```python
from build123d import *

# Parameters (mm, degrees)
SKETCH1_W           = 50
SKETCH1_H           = 170
BOSS_EXTRUDE1_DEPTH = 55
SKETCH2_W           = 34
SKETCH2_H           = 27
CUT_EXTRUDE1_DEPTH  = 181.416185527
SKETCH3_W           = 10
SKETCH3_H           = 24
SKETCH3_R           = 4.25
SKETCH3_R_2         = 1
CUT_EXTRUDE2_DEPTH  = 186.539753153
SKETCH4_W           = 2
SKETCH4_H           = 24
CUT_EXTRUDE3_DEPTH  = 178.623196683
SKETCH5_W           = 6.25
SKETCH5_H           = 11.25
CUT_EXTRUDE4_DEPTH  = 186.539753153
SKETCH6_W           = 38
SKETCH6_H           = 10
CUT_EXTRUDE5_DEPTH  = 181.416185527
SKETCH8_W           = 13.25
SKETCH8_H           = 2.25
CUT_EXTRUDE7_DEPTH  = 186.539753153
SKETCH9_W           = 34
SKETCH9_H           = 35.25
CUT_EXTRUDE8_DEPTH  = 179.297679458
SKETCH11_W          = 13.25
SKETCH11_H          = 20.25
CUT_EXTRUDE9_DEPTH  = 184.480414486
SKETCH12_W          = 28.5
SKETCH12_H          = 15
BOSS_EXTRUDE2_DEPTH = 8
SKETCH14_W          = 34
SKETCH14_H          = 15
SKETCH14_H_2        = 10.25
BOSS_EXTRUDE3_DEPTH = 13.25
SKETCH16_R          = 4.5
SKETCH16_R_2        = 2.5
CUT_EXTRUDE13_DEPTH = 8
SKETCH17_R          = 4.5
SKETCH17_W          = 55
SKETCH17_H          = 10.25
CUT_EXTRUDE15_DEPTH = 175.384811552
SKETCH18_W          = 71.25
SKETCH18_H          = 27.5
SKETCH18_W_2        = 13.75
SKETCH18_W_3        = 16.25
BOSS_EXTRUDE4_DEPTH = 50


with BuildPart() as part:
    # Sketch1 → Boss-Extrude1 (new body)
    with BuildSketch(Plane.XY):
        with Locations((0, -85)):
            Rectangle(SKETCH1_W, SKETCH1_H)
    extrude(amount=-BOSS_EXTRUDE1_DEPTH)

    # Sketch2 → Cut-Extrude1 (cut, through all)
    with BuildSketch(Plane.XY):
        with Locations((0, -13.5)):
            Rectangle(SKETCH2_W, SKETCH2_H)
    extrude(amount=-CUT_EXTRUDE1_DEPTH, mode=Mode.SUBTRACT)

    # Sketch3 → Cut-Extrude2 (cut, through all)
    with BuildSketch(Plane(origin=(25, 0, 0), x_dir=(0, 0, -1), z_dir=(1, 0, 0))):
        with Locations((50, -12)):
            Rectangle(SKETCH3_W, SKETCH3_H)
        with Locations((5, -12)):
            Rectangle(SKETCH3_W, SKETCH3_H)
        with Locations(Location((27.5, -12.75, 0), (0, 0, 90))):
            Circle(SKETCH3_R)
        with Locations(Location((35.5, -12.75, 0), (0, 0, 90))):
            Circle(SKETCH3_R_2)
        with Locations(Location((27.5, -4.75, 0), (0, 0, 90))):
            Circle(SKETCH3_R_2)
        with Locations(Location((27.5, -20.75, 0), (0, 0, 90))):
            Circle(SKETCH3_R_2)
        with Locations(Location((19.5, -12.75, 0), (0, 0, 90))):
            Circle(SKETCH3_R_2)
    extrude(amount=-CUT_EXTRUDE2_DEPTH, mode=Mode.SUBTRACT)

    # Sketch4 → Cut-Extrude3 (cut, through all)
    with BuildSketch(Plane.XY.offset(-10)):
        with Locations((-18, -12)):
            Rectangle(SKETCH4_W, SKETCH4_H)
        with Locations((18, -12)):
            Rectangle(SKETCH4_W, SKETCH4_H)
    extrude(amount=-CUT_EXTRUDE3_DEPTH, mode=Mode.SUBTRACT)

    # Sketch5 → Cut-Extrude4 (cut, through all)
    with BuildSketch(Plane(origin=(25, 0, 0), x_dir=(0, 0, -1), z_dir=(1, 0, 0))):
        with BuildLine():
            Line((45, 0), (10, 0))
            Line((10, 0), (10, -12.75))
            Line((10, -12.75), (16.25, -12.75))
            ThreePointArc((16.25, -12.75), (27.5, -1.5), (38.75, -12.75))
            Line((38.75, -12.75), (45, -12.75))
            Line((45, -12.75), (45, 0))
        make_face()
        with Locations((13.125, -18.375)):
            Rectangle(SKETCH5_W, SKETCH5_H)
        with Locations((41.875, -18.375)):
            Rectangle(SKETCH5_W, SKETCH5_H)
    extrude(amount=-CUT_EXTRUDE4_DEPTH, mode=Mode.SUBTRACT)

    # Sketch6 → Cut-Extrude5 (cut, through all)
    with BuildSketch(Plane.XY):
        with Locations((0, -29)):
            Rectangle(SKETCH6_W, SKETCH6_H)
    extrude(amount=-CUT_EXTRUDE5_DEPTH, mode=Mode.SUBTRACT)

    # Sketch8 → Cut-Extrude7 (cut, through all)
    with BuildSketch(Plane(origin=(25, 0, 0), x_dir=(0, 0, -1), z_dir=(1, 0, 0))):
        with BuildLine():
            Line((27.5, -157.5), (27.5, -132.5))
            Line((27.5, -132.5), (13.25, -132.5))
            Line((13.25, -132.5), (13.25, -167.75))
            Line((13.25, -167.75), (17.25, -167.75))
            ThreePointArc((17.25, -167.75), (20.252155493, -160.502155493), (27.5, -157.5))
        make_face()
        with BuildLine():
            Line((41.75, -167.75), (41.75, -132.5))
            Line((41.75, -132.5), (27.5, -132.5))
            Line((27.5, -132.5), (27.5, -157.5))
            ThreePointArc((27.5, -157.5), (34.747844507, -160.502155493), (37.75, -167.75))
            Line((37.75, -167.75), (41.75, -167.75))
        make_face()
        with Locations((48.375, -168.875)):
            Rectangle(SKETCH8_W, SKETCH8_H)
        with Locations((6.625, -168.875)):
            Rectangle(SKETCH8_W, SKETCH8_H)
        with BuildLine():
            Line((17.25, -167.75), (13.25, -167.75))
            Line((13.25, -167.75), (13.25, -170))
            Line((13.25, -170), (17.5, -170))
            ThreePointArc((17.5, -170), (17.31269172, -168.881923142), (17.25, -167.75))
        make_face()
        with BuildLine():
            Line((41.75, -170), (41.75, -167.75))
            Line((41.75, -167.75), (37.75, -167.75))
            ThreePointArc((37.75, -167.75), (37.68730828, -168.881923142), (37.5, -170))
            Line((37.5, -170), (41.75, -170))
        make_face()
        with BuildLine():
            Line((27.5, -167.75), (27.5, -157.5))
            ThreePointArc((27.5, -157.5), (20.252155493, -160.502155493), (17.25, -167.75))
            Line((17.25, -167.75), (27.5, -167.75))
        make_face()
        with BuildLine():
            ThreePointArc((37.75, -167.75), (34.747844507, -160.502155493), (27.5, -157.5))
            Line((27.5, -157.5), (27.5, -167.75))
            Line((27.5, -167.75), (37.75, -167.75))
        make_face()
        with BuildLine():
            Line((27.5, -170), (27.5, -167.75))
            Line((27.5, -167.75), (17.25, -167.75))
            ThreePointArc((17.25, -167.75), (17.31269172, -168.881923142), (17.5, -170))
            Line((17.5, -170), (27.5, -170))
        make_face()
        with BuildLine():
            ThreePointArc((37.5, -170), (37.68730828, -168.881923142), (37.75, -167.75))
            Line((37.75, -167.75), (27.5, -167.75))
            Line((27.5, -167.75), (27.5, -170))
            Line((27.5, -170), (37.5, -170))
        make_face()
    extrude(amount=-CUT_EXTRUDE7_DEPTH, mode=Mode.SUBTRACT)

    # Sketch9 → Cut-Extrude8 (cut, through all)
    with BuildSketch(Plane.XY):
        with Locations((0, -150.125)):
            Rectangle(SKETCH9_W, SKETCH9_H)
    extrude(amount=-CUT_EXTRUDE8_DEPTH, mode=Mode.SUBTRACT)

    # Sketch11 → Cut-Extrude9 (cut, through all)
    with BuildSketch(Plane(origin=(25, 0, 0), x_dir=(0, 0, -1), z_dir=(1, 0, 0))):
        with BuildLine():
            ThreePointArc((17.25, -167.75), (20.252155493, -160.502155493), (27.5, -157.5))
            Line((27.5, -157.5), (27.5, -147.5))
            Line((27.5, -147.5), (13.25, -147.5))
            Line((13.25, -147.5), (13.25, -167.75))
            Line((13.25, -167.75), (17.25, -167.75))
        make_face()
        with BuildLine():
            Line((27.5, -147.5), (27.5, -157.5))
            ThreePointArc((27.5, -157.5), (34.747844507, -160.502155493), (37.75, -167.75))
            Line((37.75, -167.75), (41.75, -167.75))
            Line((41.75, -167.75), (41.75, -147.5))
            Line((41.75, -147.5), (27.5, -147.5))
        make_face()
        with Locations((48.375, -157.625)):
            Rectangle(SKETCH11_W, SKETCH11_H)
        with Locations((6.625, -157.625)):
            Rectangle(SKETCH11_W, SKETCH11_H)
    extrude(amount=-CUT_EXTRUDE9_DEPTH, mode=Mode.SUBTRACT)

    # Sketch12 → Boss-Extrude2 (add)
    with BuildSketch(Plane(origin=(25, 0, 0), x_dir=(0, 0, -1), z_dir=(1, 0, 0))):
        with Locations((27.5, -140)):
            Rectangle(SKETCH12_W, SKETCH12_H)
    boss_extrude2 = extrude(amount=-BOSS_EXTRUDE2_DEPTH)

    # Mirror1: Boss-Extrude2 across plane
    add(boss_extrude2.mirror(Plane(origin=(0, 0, 0), x_dir=(0, 0, 1), z_dir=(1, 0, 0))))

    # Sketch14 → Boss-Extrude3 (add)
    with BuildSketch(Plane.XY):
        with Locations((0, -140)):
            Rectangle(SKETCH14_W, SKETCH14_H)
        with Locations((0, -152.625)):
            Rectangle(SKETCH14_W, SKETCH14_H_2)
    boss_extrude3 = extrude(amount=-BOSS_EXTRUDE3_DEPTH)

    # Mirror2: Boss-Extrude3 across plane
    add(boss_extrude3.mirror(Plane.XY.offset(-27.5)))

    # Sketch16 → Cut-Extrude13 (cut)
    # profile 1 of 3: a face of its own
    with BuildSketch(Plane(origin=(25, 0, 0), x_dir=(0, 0, -1), z_dir=(1, 0, 0))):
        with Locations(Location((16.5, -135.75, 0), (0, 0, 90))):
            Circle(SKETCH16_R)
        with Locations((16.5, -135.75)):
            Circle(SKETCH16_R_2, mode=Mode.SUBTRACT)
    # profile 2 of 3: a face of its own
    with BuildSketch(Plane(origin=(25, 0, 0), x_dir=(0, 0, -1), z_dir=(1, 0, 0))):
        with Locations((16.5, -135.75)):
            Circle(SKETCH16_R_2)
    # profile 3 of 3: a face of its own
    with BuildSketch(Plane(origin=(25, 0, 0), x_dir=(0, 0, -1), z_dir=(1, 0, 0))):
        with Locations(Location((38.5, -135.75, 0), (0, 0, 90))):
            Circle(SKETCH16_R)
    cut_extrude13 = extrude(amount=-CUT_EXTRUDE13_DEPTH, mode=Mode.SUBTRACT)

    # Mirror3: Cut-Extrude13 across plane
    add(cut_extrude13.mirror(Plane(origin=(0, 0, 0), x_dir=(0, 0, 1), z_dir=(1, 0, 0))), mode=Mode.SUBTRACT)

    # Sketch17 → Cut-Extrude15 (cut, through all)
    # profile 1 of 4: a face of its own
    with BuildSketch(Plane(origin=(25, 0, 0), x_dir=(0, 0, -1), z_dir=(1, 0, 0))):
        Polygon((55, -51.5), (27.5, -51.5), (0, -51.5), (0, -147.5), (55, -147.5), align=None)
        with Locations((16.5, -135.75)):
            Circle(SKETCH17_R, mode=Mode.SUBTRACT)
        with Locations((38.5, -135.75)):
            Circle(SKETCH17_R, mode=Mode.SUBTRACT)
    # profile 2 of 4: a face of its own
    with BuildSketch(Plane(origin=(25, 0, 0), x_dir=(0, 0, -1), z_dir=(1, 0, 0))):
        with Locations((27.5, -152.625)):
            Rectangle(SKETCH17_W, SKETCH17_H)
    # profile 3 of 4: a face of its own
    with BuildSketch(Plane(origin=(25, 0, 0), x_dir=(0, 0, -1), z_dir=(1, 0, 0))):
        with Locations((38.5, -135.75)):
            Circle(SKETCH17_R)
    # profile 4 of 4: a face of its own
    with BuildSketch(Plane(origin=(25, 0, 0), x_dir=(0, 0, -1), z_dir=(1, 0, 0))):
        with Locations((16.5, -135.75)):
            Circle(SKETCH17_R)
    extrude(amount=-CUT_EXTRUDE15_DEPTH, mode=Mode.SUBTRACT)

    # Sketch18 → Boss-Extrude4 (add)
    with BuildSketch(Plane(origin=(25, 0, 0), x_dir=(0, 0, -1), z_dir=(1, 0, 0))):
        with Locations((-35.625, -37.75)):
            Rectangle(SKETCH18_W, SKETCH18_H)
        with Locations((61.875, -37.75)):
            Rectangle(SKETCH18_W_2, SKETCH18_H)
        Polygon((38.75, -51.5), (38.75, -24), (16.25, -24), (0, -24), (0, -51.5), align=None)
        with Locations((46.875, -37.75)):
            Rectangle(SKETCH18_W_3, SKETCH18_H)
    extrude(amount=-BOSS_EXTRUDE4_DEPTH)


solid = part.part
```
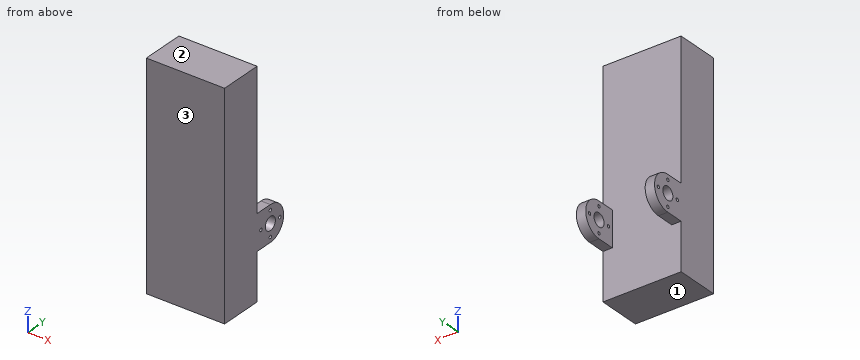
Build history of the part. All positions in model axes, mm. Face numbers are marked on the shaded views. Round coordinates to 2 decimals unless told otherwise and drop trailing zeros. Order: outer loops, then holes, each group sorted by start corner. A loop starts at its lowest first (then second) coordinate and runs counter-clockwise, first axis right, second up. Notation, with made-up numbers: (70, -27.75) -> (123, -27.75) arc R20 cw to (123, -23.75) -> close; hole circle Ø7 at (-2, 78). An arc over 180 degrees is marked (long way). Answer in a Markdown table with one row per item.
1) Band-saw the part on A-A on x = -12.5. Give the cut face in (y, z), and give its area (3 significant figures).
Values:
| item | result |
|---|---|
| outline | (-51.5, -68.75) -> (-24, -68.75) -> (-24, 71.25) -> (-51.5, 71.25) -> close |
| area | 3,850 mm2 |
2) Wall check: L1, parallel to Z at x = 20.65, y = -12.75; L2, parallel to Z at x = -22, y = -12; L3, parallel to Y at x = 21, z = -27. Give the ranges that are in metal, low to high.
Values:
| item | result |
|---|---|
| L1 | -38.75 to -36.5, -34.5 to -31.75, -23.25 to -20.5, -18.5 to -16.25 |
| L2 | -38.72 to -36.16, -34.84 to -31.68, -23.32 to -20.16, -18.84 to -16.28 |
| L3 | -51.5 to -21.62, -19.88 to -16.97, -8.53 to -5.62, -3.88 to -1.51 |
3) Mould opens along Z. For the marked faces 1, 2 and 3 say: released by +Z, released by -Z, zero draft, split by the parting line, or undercut.
Values:
| item | result |
|---|---|
| face 1 | released by -Z |
| face 2 | released by +Z |
| face 3 | zero draft |
4) Band-saw the part on B-B on z = 7. Give the cut face in (x, y), and give its area (4 significant figures).
Values:
| item | result |
|---|---|
| outline | (-25, -51.5) -> (25, -51.5) -> (25, -24) -> (-25, -24) -> close |
| area | 1,375 mm2 |
5) Pin check, flat tips, straight feed: P1, Ø2.5, axis at y = -4.75, z = -27.5, coming from the +X side; P2, Ø4, axis at x = -19.5, y = -9.5, coming from the -Z side; P3, Ø3, axis at x = 21, y = -20, coming from the -Z side; P4, Ø1.8, axis at x = -22.5, y = -20, coming from the +Z side. Stop position of each tip, or through.
Values:
| item | result |
|---|---|
| P1 | x = 25 |
| P2 | z = -38.68 |
| P3 | z = -38.75 |
| P4 | z = -16.25 |
